Can you work these out from the drawing? Everything is in mm from the part's minimum corner. Coordinates: 2 decimals unless noted, no trailing zeros. Order: outer loops, then holes, each group sorted by start corner. A loop starts at its lowest first (then second) coordinate and runs counter-clockwise, first axis right, second up. Notation, with made-up numbers: (79.25, 33) - (113.25, 33) arc R19 cw to (113.25, 58) - close; hole circle Ø7 at (80, 78). An arc over 180 degrees is marked (long way). Use a Markdown table: item, result. Add a question column.
(1) If I drill on L1, parallel to Y at x = 154, z = 2.1; L2, parallel to X at y = 16, z = 2.1, over which ranges is the centre line in solid material (lowest first)? Write a range as [from, to].
(2) I want a section at B-B (z = 0.95). List the corners of the cut face in (x, y) for me.
(3) I want a section at A-A (y = 198.5). List the corners of the cut face in (x, z) for me, and give its area (3 significant figures).
(4) For pin 1 Ø2.5 at (y, z) = (12, 3.5) entering from -X, with a flat end and sliding along its axis, tell me the tip position at first contact or that it passes through.
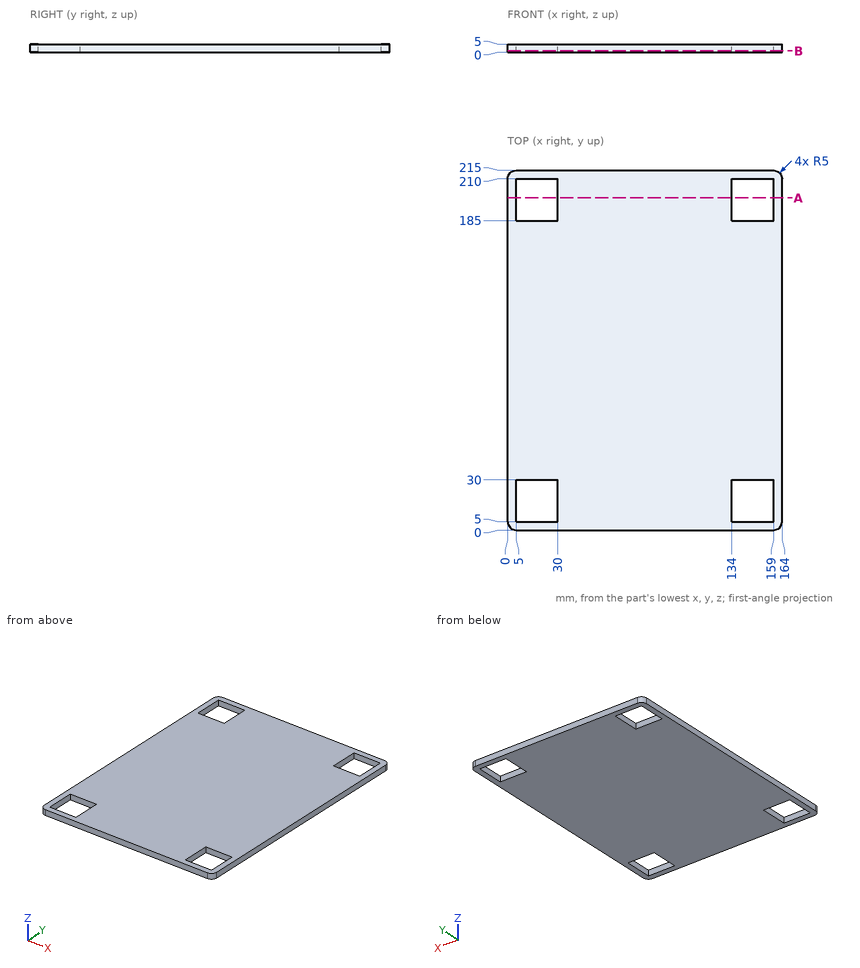
Answers follow:
| question | item | result |
|---|---|---|
| 1 | L1 | y = [0, 5], [30, 185], [210, 215] |
| 1 | L2 | x = [0, 5], [30, 134], [159, 164] |
| 2 | outline | (0, 5) arc R5 ccw to (5, 0) - (159, 0) arc R5 ccw to (164, 5) - (164, 210) arc R5 ccw to (159, 215) - (5, 215) arc R5 ccw to (0, 210) - close; hole (5, 5) - (30, 5) - (30, 30) - (5, 30) - close; hole (5, 185) - (30, 185) - (30, 210) - (5, 210) - close; hole (134, 5) - (159, 5) - (159, 30) - (134, 30) - close; hole (134, 185) - (159, 185) - (159, 210) - (134, 210) - close |
| 3 | outline | (0, 0) - (5, 0) - (5, 5) - (0, 5) - close; (30, 0) - (134, 0) - (134, 5) - (30, 5) - close; (159, 0) - (164, 0) - (164, 5) - (159, 5) - close |
| 3 | area | 570 mm² |
| 4 | pin 1 | stops at x = 0 |
